```python
from build123d import *

# Parameters (mm, degrees)
SKETCH1_W           = 50
SKETCH1_H           = 50
BOSS_EXTRUDE1_DEPTH = 10
SKETCH3_W           = 1.37
SKETCH3_H           = 6.568764243
CUT_EXTRUDE1_DEPTH  = 50
LPATTERN1_COUNT     = 7
LPATTERN1_PITCH     = 6


with BuildPart() as part:
    # Sketch1 → Boss-Extrude1 (new body)
    with BuildSketch(Plane(origin=(0, 0, 0), x_dir=(1, 0, 0), z_dir=(0, 1, 0))):
        with Locations((25, -25)):
            Rectangle(SKETCH1_W, SKETCH1_H)
    extrude(amount=BOSS_EXTRUDE1_DEPTH)

    # Sketch3 → Cut-Extrude1 (cut)
    with BuildSketch(Plane.XY.offset(50)):
        with Locations((7.015961915, 3.284382122)):
            Rectangle(SKETCH3_W, SKETCH3_H)
    cut_extrude1 = extrude(amount=-CUT_EXTRUDE1_DEPTH, mode=Mode.SUBTRACT)

    # LPattern1: Cut-Extrude1 ×7
    with Locations(*[(i * LPATTERN1_PITCH, 0, 0) for i in range(1, LPATTERN1_COUNT)]):
        add(cut_extrude1, mode=Mode.SUBTRACT)


solid = part.part
```
Geometry: final body of the model. Coordinates: model frame, mm. A direction names the side the tool comes from. Round coordinates to 2 decimals unless told otherwise and drop trailing zeros. Order: outer loops, then holes, each group sorted by start corner. A loop starts at its lowest first (then second) coordinate and runs counter-clockwise, first axis right, second up. Notation, with made-up numbers: (-25.75, 84.5) -> (9.25, 84.5) arc R16 ccw to (9.25, 93.5) -> close; hole circle Ø3 at (15, -5.75). An arc over 180 degrees is marked (long way). Write each question's results on one line, items separated by ' | '.
Q1. Section query C-C (x = 43). Output: boundary loops of the cut face in (y, z).
Response values:
outline: (6.57, 0) -> (10, 0) -> (10, 50) -> (6.57, 50) -> close
Q2. Ray query, line 1 along Y through (x, z) = (31, 20). Return the intervals inside material, ascending.
Response values:
line 1: 6.57 to 10
Q3. Access query for faces 1 (the face through (7, 6.569, 25)), 2 (the face through (22, 0, 25)). Directions: +Z, -Z, +X, -X, +Y, -Y. A direction counts if a zero-diameter tool reaches every point of the face in a straight line with its end or side. Return the directions, or none.
Response values:
face 1: +Z, -Z, -Y | face 2: +Z, -Z, +X, -X, -Y
Q4. Pin query (flat end, axial travel): pin 1 Ø1.1 at (x, z) = (19, 28.5) entering from -Y. Return the tip coordinate at first contact, or that it passes through.
Response values:
pin 1: y = 6.57
Q5. Section query A-A (y = 5.25). Count the separate pieces of the cut face and the enclosed holes in it, and give its area (3 significant figures).
Response values:
separate pieces: 8 | enclosed holes: 0 | area: 2,020 mm²
Q6. Pull-direction query (X, two-part tool) for faces 3 (the face through (50, 5, 25)), 4 (the face through (25, 7, 50)), 5 (the face through (13.701, 3, 25)); classes: released by +X, released by -X, zero draft, split by the parting line, or undercut.
Response values:
face 3: released by +X | face 4: zero draft | face 5: undercut
